The listing builds one solid part. Answer for the finished solid, in the listing's coordinates (mm). A direction names the side the tool comes from. Coordinates: 2 decimals unless noted, no trailing zeros. Loops run counter-clockwise (first coordinate to the right, second up) from the corner with the lowest first, then second, coordinate; pieces in that order, holes last. Notation, with made-up numbers: M -11,-6.5 L 36,-6.5 A17 cw 36,16.5 Z; hole C -34.75,59 d2. An arc over 180 degrees is marked long. Answer as CSV lines item,"result". Start each with the question number.
```python
from build123d import *

# Parameters (mm, degrees)
SKETCH1_W           = 21.082
SKETCH1_H           = 43.18
BOSS_EXTRUDE1_DEPTH = 2.5
SKETCH2_R           = 1.4
BOSS_EXTRUDE2_DEPTH = 5


with BuildPart() as part:
    # Sketch1 → Boss-Extrude1 (new body)
    with BuildSketch(Plane(origin=(0, 0, 0), x_dir=(1, 0, 0), z_dir=(0, 1, 0))):
        Rectangle(SKETCH1_W, SKETCH1_H)
    extrude(amount=BOSS_EXTRUDE1_DEPTH)

    # Sketch2 → Boss-Extrude2 (add)
    # profile 1 of 2: a face of its own
    with BuildSketch(Plane(origin=(0, 2.5, 0), x_dir=(1, 0, 0), z_dir=(0, 1, 0))):
        with BuildLine():
            Line((10.541, 12.304485913), (10.541, 18.675514087))
            ThreePointArc((10.541, 18.675514087), (4.391, 15.49), (10.541, 12.304485913))
        make_face()
        with Locations(Location((8.291, 15.49, 0), (0, 0, 270))):
            Circle(SKETCH2_R, mode=Mode.SUBTRACT)
    # profile 2 of 2: a face of its own
    with BuildSketch(Plane(origin=(0, 2.5, 0), x_dir=(1, 0, 0), z_dir=(0, 1, 0))):
        with BuildLine():
            ThreePointArc((-10.541, -18.675514087), (-4.391, -15.49), (-10.541, -12.304485913))
            Line((-10.541, -12.304485913), (-10.541, -18.675514087))
        make_face()
        with Locations(Location((-8.291, -15.49, 0), (0, 0, 270))):
            Circle(SKETCH2_R, mode=Mode.SUBTRACT)
    extrude(amount=BOSS_EXTRUDE2_DEPTH)


solid = part.part
```
Item 1: Each of these flat-tipped pins is pushed along its axis until it touches: P1, Ø1, axis at x = 8, y = 6.5, coming from the -Z side; P2, Ø6.5, axis at x = 5, z = 10, coming from the +Y side; P3, Ø2, axis at x = 8, y = 4, coming from the +Z side; P4, Ø3, axis at y = 5, z = 7, coming from the +X side. Where does it stop, or does it pass through?
Item 2: Section D-D on x = -6 is taken. Determine the outline of the cut face in (y, z).
Item 3: Consider line 1 (Y direction, x = -6.5, z = -17.5); line 2 (Z direction, x = -8, y = 7); line 3 (Z direction, x = 7.5, y = 5.5). Determine where each line is inside the solid, lowest interval first.
Item 4: For a pull along X with two mould halves and no side action, classify faces 3 (the face through (-10.541, 2, 5)), 4 (the face through (0, 1, -21.59)), 5 (the face through (-8, 2.5, 15)), 6 (the face through (8, 2.5, -16)) as pulls with the +X half, pulls with the -X half, needs draft (parallel to the pull), parting line crosses it, or undercut.
Item 5: Section A-A on y = 5 is taken. Determine the outline of the cut face in (x, z).
Item 6: Section B-B on x = -8.75 is taken. Determine the outline of the cut face in (y, z), then the cut area to 3 significant figures.
Item 7: Section C-C on z = -15.49 is taken. Determine the outline of the cut face in (x, y).
Item 8: For faces 1 (the face through (10.541, 2, -4)), 2 (the face through (-4.393, 4.965, 15.609)), determine the directions among +Z, -Z, +X, -X, +Y, -Y from which every point of the face is accessible in a straight line to the end or side of a thin tool.
Results are:
1,P1,"z = -19.39"
1,P2,"y = 2.5"
1,P3,"z = -11.59"
1,P4,"through"
2,outline,"M 0,-21.59 L 2.5,-21.59 L 2.5,12.33 L 7.5,12.33 L 7.5,18.65 L 2.5,18.65 L 2.5,21.59 L 0,21.59 Z"
3,line 1,"0 to 2.5"
3,line 2,"11.6 to 14.12, 16.86 to 19.38"
3,line 3,"-19.31 to -16.65, -14.33 to -11.67"
4,face 3,"pulls with the -X half"
4,face 4,"needs draft"
4,face 5,"undercut"
4,face 6,"undercut"
5,outline,"M -10.54,12.3 A3.9 ccw long -10.54,18.68 Z; M 10.54,-18.68 L 10.54,-12.3 A3.9 ccw long Z; hole C -8.29,15.49 d2.8; hole C 8.29,-15.49 d2.8"
6,outline,"M 0,-21.59 L 2.5,-21.59 L 2.5,11.62 L 7.5,11.62 L 7.5,14.17 L 2.5,14.17 L 2.5,16.81 L 7.5,16.81 L 7.5,19.36 L 2.5,19.36 L 2.5,21.59 L 0,21.59 Z"
6,area,"133 mm²"
7,outline,"M -10.54,0 L 10.54,0 L 10.54,7.5 L 9.69,7.5 L 9.69,2.5 L 6.89,2.5 L 6.89,7.5 L 4.39,7.5 L 4.39,2.5 L -10.54,2.5 Z"
8,face 1,"+Z, -Z, +X, +Y, -Y"
8,face 2,"+Y"
